Work out the finished part from the listing and answer in its coordinate system (mm). Give positions to 0.01 mm unless a question says otherwise; leave off trailing zeros. Loops run counter-clockwise (first coordinate to the right, second up) from the corner with the lowest first, then second, coordinate; pieces in that order, holes last. Notation, with made-up numbers: (45, -0.75) - (91, -0.75) arc R25 ccw to (91, 25.25) - close; hole circle Ø4 at (22.5, 38.5). An arc over 180 degrees is marked (long way). One line per item, written item: value.
from build123d import *

# Parameters (mm, degrees)
SKETCH1_W           = 31
SKETCH1_H           = 61
BOSS_EXTRUDE1_DEPTH = 25
SKETCH2_R           = 1.75
BOSS_EXTRUDE2_DEPTH = 10
FILLET1_R           = 2


with BuildPart() as part:
    # Sketch1 → Boss-Extrude1 (new body)
    with BuildSketch(Plane(origin=(0, 0, 0), x_dir=(1, 0, 0), z_dir=(0, 1, 0))):
        Rectangle(SKETCH1_W, SKETCH1_H)
    extrude(amount=BOSS_EXTRUDE1_DEPTH)

    # Sketch2 → Boss-Extrude2 (add)
    with BuildSketch(Plane.XY.offset(30.5)):
        with Locations(Location((13.5, 14.5, 0), (0, 0, 180))):
            Circle(SKETCH2_R)
        with Locations((13.5, 10.5)):
            Circle(SKETCH2_R)
    extrude(amount=BOSS_EXTRUDE2_DEPTH)

    # Fillet1
    # the kernel refuses this fillet: 2 mm, written as the material it takes off along each edge
    with BuildSketch(Plane(origin=(-13.5, 23, 28.5), x_dir=(0, 1, 0), z_dir=(-1, 0, 0))) as fillet1_piece_1_section:
        Polygon((0, 0), (FILLET1_R, 0), (FILLET1_R, -FILLET1_R), (0, -FILLET1_R), align=None)
    fillet1_piece_1 = extrude(amount=FILLET1_R, mode=Mode.PRIVATE)
    fillet1_piece_1 = fillet1_piece_1 - Plane(origin=(-13.5, 23, 28.5), x_dir=(0, -0.7071067811865475, -0.7071067811865475), z_dir=(-1, 0, 0)) * Sphere(FILLET1_R, mode=Mode.PRIVATE)
    add(fillet1_piece_1, mode=Mode.SUBTRACT)
    with BuildSketch(Plane(origin=(-13.5, 23, -28.5), x_dir=(-1, 0, 0), z_dir=(0, 0, -1))) as fillet1_piece_2_section:
        Polygon((0, 0), (FILLET1_R, 0), (FILLET1_R, FILLET1_R), (0, FILLET1_R), align=None)
    fillet1_piece_2 = extrude(amount=FILLET1_R, mode=Mode.PRIVATE)
    fillet1_piece_2 = fillet1_piece_2 - Plane(origin=(-13.5, 23, -28.5), x_dir=(0.7071067811865475, -0.7071067811865475, 0), z_dir=(0, 0, -1)) * Sphere(FILLET1_R, mode=Mode.PRIVATE)
    add(fillet1_piece_2, mode=Mode.SUBTRACT)
    with BuildSketch(Plane(origin=(13.5, 23, 28.5), x_dir=(0, 1, 0), z_dir=(1, 0, 0))) as fillet1_piece_3_section:
        Polygon((0, 0), (FILLET1_R, 0), (FILLET1_R, FILLET1_R), (0, FILLET1_R), align=None)
    fillet1_piece_3 = extrude(amount=FILLET1_R, mode=Mode.PRIVATE)
    fillet1_piece_3 = fillet1_piece_3 - Plane(origin=(13.5, 23, 28.5), x_dir=(0, -0.7071067811865475, -0.7071067811865475), z_dir=(1, 0, 0)) * Sphere(FILLET1_R, mode=Mode.PRIVATE)
    add(fillet1_piece_3, mode=Mode.SUBTRACT)
    with BuildSketch(Plane(origin=(13.5, 23, -28.5), x_dir=(1, 0, 0), z_dir=(0, 0, -1))) as fillet1_piece_4_section:
        Polygon((0, 0), (FILLET1_R, 0), (FILLET1_R, -FILLET1_R), (0, -FILLET1_R), align=None)
    fillet1_piece_4 = extrude(amount=FILLET1_R, mode=Mode.PRIVATE)
    fillet1_piece_4 = fillet1_piece_4 - Plane(origin=(13.5, 23, -28.5), x_dir=(-0.7071067811865475, -0.7071067811865475, 0), z_dir=(0, 0, -1)) * Sphere(FILLET1_R, mode=Mode.PRIVATE)
    add(fillet1_piece_4, mode=Mode.SUBTRACT)
    with BuildSketch(Plane(origin=(13.5, 2, 28.5), x_dir=(0, -1, 0), z_dir=(1, 0, 0))) as fillet1_piece_5_section:
        Polygon((0, 0), (FILLET1_R, 0), (FILLET1_R, -FILLET1_R), (0, -FILLET1_R), align=None)
    fillet1_piece_5 = extrude(amount=FILLET1_R, mode=Mode.PRIVATE)
    fillet1_piece_5 = fillet1_piece_5 - Plane(origin=(13.5, 2, 28.5), x_dir=(0, 0.7071067811865475, -0.7071067811865475), z_dir=(1, 0, 0)) * Sphere(FILLET1_R, mode=Mode.PRIVATE)
    add(fillet1_piece_5, mode=Mode.SUBTRACT)
    with BuildSketch(Plane(origin=(-13.5, 2, 28.5), x_dir=(0, -1, 0), z_dir=(-1, 0, 0))) as fillet1_piece_6_section:
        Polygon((0, 0), (FILLET1_R, 0), (FILLET1_R, FILLET1_R), (0, FILLET1_R), align=None)
    fillet1_piece_6 = extrude(amount=FILLET1_R, mode=Mode.PRIVATE)
    fillet1_piece_6 = fillet1_piece_6 - Plane(origin=(-13.5, 2, 28.5), x_dir=(0, 0.7071067811865475, -0.7071067811865475), z_dir=(-1, 0, 0)) * Sphere(FILLET1_R, mode=Mode.PRIVATE)
    add(fillet1_piece_6, mode=Mode.SUBTRACT)
    with BuildSketch(Plane(origin=(-13.5, 2, -28.5), x_dir=(-1, 0, 0), z_dir=(0, 0, -1))) as fillet1_piece_7_section:
        Polygon((0, 0), (FILLET1_R, 0), (FILLET1_R, -FILLET1_R), (0, -FILLET1_R), align=None)
    fillet1_piece_7 = extrude(amount=FILLET1_R, mode=Mode.PRIVATE)
    fillet1_piece_7 = fillet1_piece_7 - Plane(origin=(-13.5, 2, -28.5), x_dir=(0.7071067811865475, 0.7071067811865475, 0), z_dir=(0, 0, -1)) * Sphere(FILLET1_R, mode=Mode.PRIVATE)
    add(fillet1_piece_7, mode=Mode.SUBTRACT)
    with BuildSketch(Plane(origin=(13.5, 2, -28.5), x_dir=(1, 0, 0), z_dir=(0, 0, -1))) as fillet1_piece_8_section:
        Polygon((0, 0), (FILLET1_R, 0), (FILLET1_R, FILLET1_R), (0, FILLET1_R), align=None)
    fillet1_piece_8 = extrude(amount=FILLET1_R, mode=Mode.PRIVATE)
    fillet1_piece_8 = fillet1_piece_8 - Plane(origin=(13.5, 2, -28.5), x_dir=(-0.7071067811865475, 0.7071067811865475, 0), z_dir=(0, 0, -1)) * Sphere(FILLET1_R, mode=Mode.PRIVATE)
    add(fillet1_piece_8, mode=Mode.SUBTRACT)
    with BuildSketch(Plane(origin=(-15.5, 25, 28.5), x_dir=(0, -1, 0), z_dir=(0, 0, -1)), Plane(origin=(15.5, 25, -28.5), x_dir=(0, -1, 0), z_dir=(0, 0, 1))) as fillet1_piece_9:
        with BuildLine():
            CenterArc((FILLET1_R, -FILLET1_R), FILLET1_R, 90, 90)
            Line((0, -FILLET1_R), (0, 0))
            Line((0, 0), (FILLET1_R, 0))
        make_face()
    extrude(amount=57, mode=Mode.SUBTRACT)
    with BuildSketch(Plane(origin=(13.5, 25, 30.5), x_dir=(0, 0, -1), z_dir=(-1, 0, 0)), Plane(origin=(-13.5, 0, -30.5), x_dir=(0, 1, 0), z_dir=(1, 0, 0))) as fillet1_piece_10:
        with BuildLine():
            CenterArc((FILLET1_R, FILLET1_R), FILLET1_R, 180, 90)
            Line((0, FILLET1_R), (0, 0))
            Line((0, 0), (FILLET1_R, 0))
        make_face()
    extrude(amount=27, mode=Mode.SUBTRACT)
    with BuildSketch(Plane(origin=(13.5, 0, 30.5), x_dir=(0, 0, -1), z_dir=(-1, 0, 0)), Plane(origin=(-13.5, 25, -30.5), x_dir=(0, -1, 0), z_dir=(1, 0, 0))) as fillet1_piece_11:
        with BuildLine():
            CenterArc((FILLET1_R, -FILLET1_R), FILLET1_R, 90, 90)
            Line((0, -FILLET1_R), (0, 0))
            Line((0, 0), (FILLET1_R, 0))
        make_face()
    extrude(amount=27, mode=Mode.SUBTRACT)
    with BuildSketch(Plane(origin=(-15.5, 0, 28.5), x_dir=(0, 1, 0), z_dir=(0, 0, -1)), Plane(origin=(15.5, 0, -28.5), x_dir=(0, 1, 0), z_dir=(0, 0, 1))) as fillet1_piece_12:
        with BuildLine():
            CenterArc((FILLET1_R, FILLET1_R), FILLET1_R, 180, 90)
            Line((0, FILLET1_R), (0, 0))
            Line((0, 0), (FILLET1_R, 0))
        make_face()
    extrude(amount=57, mode=Mode.SUBTRACT)
    with BuildSketch(Plane(origin=(15.5, 2, 30.5), x_dir=(0, 0, -1), z_dir=(0, 1, 0))) as fillet1_piece_13_section:
        with BuildLine():
            CenterArc((FILLET1_R, FILLET1_R), FILLET1_R, 180, 90)
            Line((0, FILLET1_R), (0, 0))
            Line((0, 0), (FILLET1_R, 0))
        make_face()
    fillet1_piece_13 = extrude(amount=21, mode=Mode.PRIVATE)
    fillet1_piece_13 = fillet1_piece_13 - Plane(origin=(13.5, 14.5, 30.013488992), x_dir=(-1, 0, 0), z_dir=(0, 0, -1)) * Cylinder(1.75, 50, mode=Mode.PRIVATE)
    fillet1_piece_13 = fillet1_piece_13 - Plane(origin=(13.5, 10.5, 30.013488992), x_dir=(1, 0, 0), z_dir=(0, 0, -1)) * Cylinder(1.75, 50, mode=Mode.PRIVATE)
    add(fillet1_piece_13, mode=Mode.SUBTRACT)
    with BuildSketch(Plane(origin=(-15.5, 2, 30.5), x_dir=(0, 0, -1), z_dir=(0, 1, 0)), Plane(origin=(-15.5, 2, -30.5), x_dir=(1, 0, 0), z_dir=(0, 1, 0))) as fillet1_piece_14:
        with BuildLine():
            CenterArc((FILLET1_R, -FILLET1_R), FILLET1_R, 90, 90)
            Line((0, -FILLET1_R), (0, 0))
            Line((0, 0), (FILLET1_R, 0))
        make_face()
    extrude(amount=21, mode=Mode.SUBTRACT)
    with BuildSketch(Plane(origin=(15.5, 2, -30.5), x_dir=(-1, 0, 0), z_dir=(0, 1, 0))) as fillet1_piece_15:
        with BuildLine():
            CenterArc((FILLET1_R, FILLET1_R), FILLET1_R, 180, 90)
            Line((0, FILLET1_R), (0, 0))
            Line((0, 0), (FILLET1_R, 0))
        make_face()
    extrude(amount=21, mode=Mode.SUBTRACT)


solid = part.part
1. A flat-ended cylindrical pin translates along its axis: pin 1 Ø1 at (x, y) = (-0.5, 16) entering from +Z. Find the tip coordinate at first contact, or state that the pin passes through.
Output:
pin 1: stops at z = 30.5
2. Find the intervals of material crossed by line 1 along Z through (x, y) = (-12, 14); line 2 along Z through (x, y) = (-12.5, 23.5); line 3 along Y through (x, z) = (-14, 9), in increasing order.
Output:
line 1: z = -30.5 to 30.5
line 2: z = -30.44 to 30.44
line 3: y = 0.06 to 24.94
3. The mould has two halves that part along Y. Classify faces 1 (the flat face through (14, 14, 40.5)), 2 (the cylindrical face through (15.25, 14.42, 34.91)), 3 (the cylindrical face through (0.19, 24.4, 29.93)): released by +Y, released by -Y, zero draft, split by the parting line, or undercut.
Output:
face 1: zero draft
face 2: undercut
face 3: released by +Y
4. Section B-B (y = 6.25) is taken. Write down the section's boundary in (x, z).
Output:
outline: (-15.5, -28.5) arc R2 ccw to (-13.5, -30.5) - (13.5, -30.5) arc R2 ccw to (15.5, -28.5) - (15.5, 28.5) arc R2 ccw to (13.5, 30.5) - (-13.5, 30.5) arc R2 ccw to (-15.5, 28.5) - close
5. Section C-C (y = 14.5) is taken. Write down the section's boundary in (x, z), and give its area (3 significant figures).
Output:
outline: (-15.5, -28.5) arc R2 ccw to (-13.5, -30.5) - (13.5, -30.5) arc R2 ccw to (15.5, -28.5) - (15.5, 28.5) arc R2 ccw to (15.25, 29.47) - (15.25, 40.5) - (11.75, 40.5) - (11.75, 30.5) - (-13.5, 30.5) arc R2 ccw to (-15.5, 28.5) - close
area: 1,920 mm²
6. Section A-A (x = 0.5) is taken. Write down the section's boundary in (y, z).
Output:
outline: (0, -28.5) arc R2 ccw to (2, -30.5) - (23, -30.5) arc R2 ccw to (25, -28.5) - (25, 28.5) arc R2 ccw to (23, 30.5) - (2, 30.5) arc R2 ccw to (0, 28.5) - close
